Answer from the drawing. Dimensions are ordinates in mm from the lowest x, y and z of the part. A direction names the side the tool comes from. Round coordinates to 2 decimals unless told otherwise and drop trailing zeros. Loops run counter-clockwise (first coordinate to the right, second up) from the corner with the lowest first, then second, coordinate; pieces in that order, holes last. Notation, with made-up numbers: (33.5, -2) - (71.5, -2) arc R20 ccw to (71.5, 11) - close; hole circle Ø4 at (27.5, 14.25). An arc over 180 degrees is marked (long way). One line per question, with ' | ' between items. Start each with the question number.
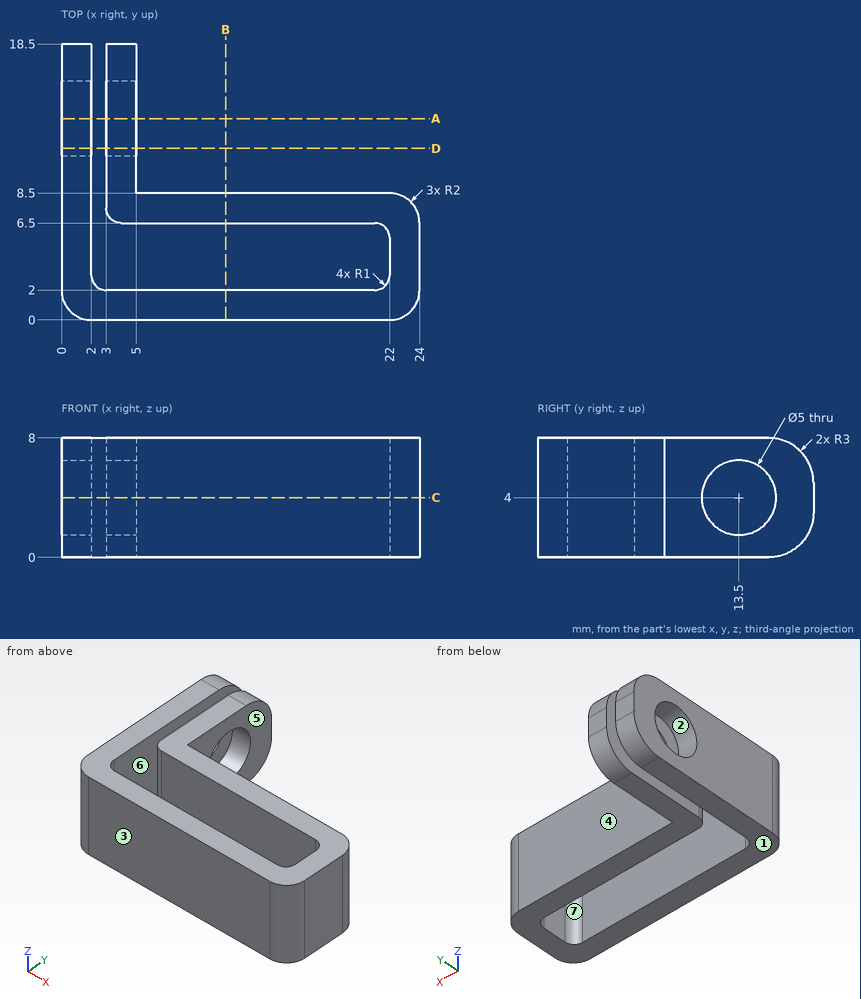
(1) Find section A-A on y = 13.5. Write down the section's boundary in (x, z), plus the area to 3 significant figures.
(2) Find section D-D on y = 11.5. Write down the section's boundary in (x, z).
(3) Find section B-B on x = 11. Write down the section's boundary in (y, z).
(4) Find section C-C on z = 4. Write down the section's boundary in (x, y).
(5) A tool of negligible diameter and unlimited length cuts with its end or side. For the marked faces 5, 6 and 7, from which of +Z, -Z, +X, -X, +Y, -Y can it reach the whole face along a straight path? Write none if from no direction.
(6) Determine the mould class of the marked faces 1, 2, 3 and 4 for opening direction Y: pulls with the +Y half, pulls with the -Y half, needs draft (parallel to the pull), parting line crosses it, or undercut.
(7) Consider L1, parallel to Z at x = 3.65, y = 13.5; L2, parallel to Y at x = 10.75, z = 5.5; L3, parallel to X at y = 9.5, z = 2.75. Determine where each line is inside the solid, lowest interval first.
(8) Each of these flat-tipped pins is pushed along its axis until it touches: P1, Ø4, axis at x = 12.5, z = 4, coming from the +Y side; P2, Ø4, axis at y = 12.5, z = 2.5, coming from the +X side. Where does it stop, or does it pass through?
Answer below:
1) outline: (0, 0) - (2, 0) - (2, 1.5) - (0, 1.5) - close; (0, 6.5) - (2, 6.5) - (2, 8) - (0, 8) - close; (3, 0) - (5, 0) - (5, 1.5) - (3, 1.5) - close; (3, 6.5) - (5, 6.5) - (5, 8) - (3, 8) - close | area: 12.0 mm2
2) outline: (0, 0) - (2, 0) - (2, 2.5) - (0, 2.5) - close; (0, 5.5) - (2, 5.5) - (2, 8) - (0, 8) - close; (3, 0) - (5, 0) - (5, 2.5) - (3, 2.5) - close; (3, 5.5) - (5, 5.5) - (5, 8) - (3, 8) - close
3) outline: (0, 0) - (2, 0) - (2, 8) - (0, 8) - close; (6.5, 0) - (8.5, 0) - (8.5, 8) - (6.5, 8) - close
4) outline: (0, 2) arc R2 ccw to (2, 0) - (22, 0) arc R2 ccw to (24, 2) - (24, 6.5) arc R2 ccw to (22, 8.5) - (5, 8.5) - (5, 11) - (3, 11) - (3, 7.5) arc R1 ccw to (4, 6.5) - (21, 6.5) arc R1 cw to (22, 5.5) - (22, 3) arc R1 cw to (21, 2) - (3, 2) arc R1 cw to (2, 3) - (2, 11) - (0, 11) - close; (0, 16) - (2, 16) - (2, 18.5) - (0, 18.5) - close; (3, 16) - (5, 16) - (5, 18.5) - (3, 18.5) - close
5) face 5: +Z, -Z, +X, +Y | face 6: +Z, -Z, +Y | face 7: +Z, -Z
6) face 1: needs draft | face 2: undercut | face 3: pulls with the -Y half | face 4: pulls with the +Y half
7) L1: 0 to 1.5, 6.5 to 8 | L2: 0 to 2, 6.5 to 8.5 | L3: 0 to 2, 3 to 5
8) P1: y = 8.5 | P2: x = 5
